Drawing for the job (mm, zero at the part's lowest x, y, z). Give positions to 0.01 mm unless a question says otherwise; leave off trailing zeros. Order: outer loops, then holes, each group sorted by start corner. A loop starts at its lowest first (then second) coordinate and runs counter-clockwise, first axis right, second up. Notation, with made-up numbers: (-6, -28.75) -> (35, -28.75) arc R14 ccw to (35, -11.75) -> close; hole circle Ø9 at (64, -10). An arc over 180 degrees is marked (long way). Use one line per item in the form item = value. Start each with the question number.
1) Cut at B-B, the plane x = 16.5. Give the cut face in (y, z).
2) Cut at C-C, the plane y = 1.85. Give the cut face in (x, z), and give its area (3 significant figures).
3) Probe line 1 (X direction, y = 2.65, z = 184); line 2 (X direction, y = 2.45, z = 97); line 3 (Z direction, x = 106.5, y = 2.5). List the from-to ranges inside material, lowest first.
4) Cut at D-D, the plane x = 78. Give the cut face in (y, z), and give its area (3 significant figures).
5) Drop flat-ended pins along their axis: P1, Ø1, axis at x = 124.5, y = 0.5, coming from the +Z side; P2, Ø1, axis at x = 81.5, z = 154.5, coming from the -Y side. Give the stop position or say it passes through.
6) Cut at A-A, the plane z = 60. Give the cut face in (x, y).
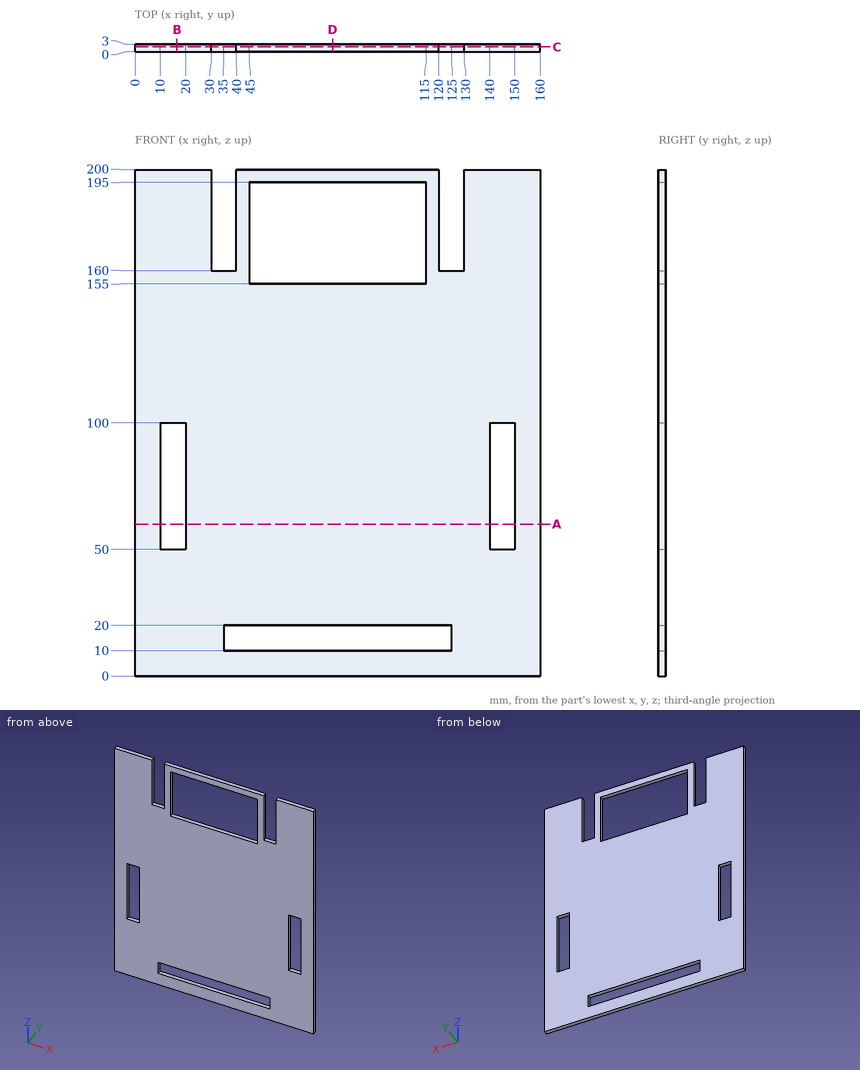
Result:
q1.outline = (0, 0) -> (3, 0) -> (3, 50) -> (0, 50) -> close; (0, 100) -> (3, 100) -> (3, 200) -> (0, 200) -> close
q2.outline = (0, 0) -> (160, 0) -> (160, 200) -> (130, 200) -> (130, 160) -> (120, 160) -> (120, 200) -> (40, 200) -> (40, 160) -> (30, 160) -> (30, 200) -> (0, 200) -> close; hole (10, 50) -> (20, 50) -> (20, 100) -> (10, 100) -> close; hole (35, 10) -> (125, 10) -> (125, 20) -> (35, 20) -> close; hole (45, 155) -> (115, 155) -> (115, 195) -> (45, 195) -> close; hole (140, 50) -> (150, 50) -> (150, 100) -> (140, 100) -> close
q2.area = 26,500 mm²
q3.line_1 = 0 to 30, 40 to 45, 115 to 120, 130 to 160
q3.line_2 = 0 to 10, 20 to 140, 150 to 160
q3.line_3 = 0 to 10, 20 to 155, 195 to 200
q4.outline = (0, 0) -> (3, 0) -> (3, 10) -> (0, 10) -> close; (0, 20) -> (3, 20) -> (3, 155) -> (0, 155) -> close; (0, 195) -> (3, 195) -> (3, 200) -> (0, 200) -> close
q4.area = 450 mm²
q5.P1 = 160
q5.P2 = 0
q6.outline = (0, 0) -> (10, 0) -> (10, 3) -> (0, 3) -> close; (20, 0) -> (140, 0) -> (140, 3) -> (20, 3) -> close; (150, 0) -> (160, 0) -> (160, 3) -> (150, 3) -> close
